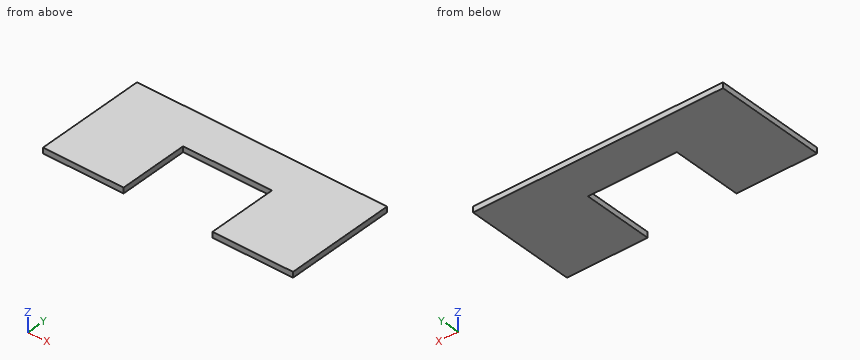
Autodesk Fusion 360 part; units mm, degrees
sketch "Sorting Mechanism Top Panel" plane through (0, 0, 0) normal (0, 0, 1) x (1, 0, 0)
  line L0 (0, 0) -> (270, 0)
  line L1 (270, 0) -> (270, 120)
  line L2 (270, 120) -> (0, 120)
  line L3 (0, 120) -> (0, 0)
  dimension "d1" = 270
  dimension "d2" = 120
extrude "Extrude1" add sketch "Sorting Mechanism Top Panel" along normal blind 6
sketch "Smartie Hopper Hole" plane through (0, 0, 6) normal (0, 0, 1) x (-1, 0, 0)
  line L0 (0, -120) -> (0, 0)
  line L1 (0, 0) -> (-270, 0)
  line L2 (-270, 0) -> (-270, -120)
  line L3 (-270, -120) -> (0, -120)
  line L4 (-87, -76) -> (-183, -76)
  line L5 (-183, -76) -> (-183, 0)
  line L6 (-183, 0) -> (-87, 0)
  line L7 (-87, 0) -> (-87, -76)
  dimension "d7" = 96
  dimension "d9" = 76
  dimension "d10" = 87
  dimension "d11" = 87
extrude "Extrude2" cut sketch "Smartie Hopper Hole" against normal blind 6 contours L1 L4 L5 L6 L7
equation "d3 = MDF_thickness"
equation "acrylic_thickness = 3 mm"
equation "MDF_thickness = 6 mm"
equation "d7 = smarties_hopper_width + 2 * acrylic_thickness"
equation "smarties_hopper_width = 90 mm"
equation "d9 = smarties_hopper_depth + 2 * acrylic_thickness"
equation "d10 = ( 270 mm - ( smarties_hopper_width + 2 * acrylic_thickness ) ) / 2"
equation "smarties_hopper_depth = 70 mm"
The model under review builds one solid part; all positions refer to its coordinate system, in mm. Round coordinates to 2 decimals unless told otherwise and drop trailing zeros. Write each loop counter-clockwise with the first axis right and the second up, starting at its lowest first coordinate (ties: lowest second). Pieces come first, ordered by that corner, then holes. Notation, with made-up numbers: M -10,0 L 39,0 A18 cw 39,30 Z; hole C -24,82.5 d7. An arc over 180 degrees is marked long. Answer as CSV lines item,"result". Start each with the question number.
Q1. Clearance check with a flat-ended pin moving along its axis: P1, Ø3, axis at x = 141.5, z = 1.5, coming from the -Y side. State where the tip first meets the part, or that it passes through.
Q2. Consider section B-B, the plane z = 3. Give the boundary of the cut face in (x, y), then the cut area to 3 significant figures.
Q3. Wall thickness on line 1 along X through (y, z) = (25.5, 4.7); line 2 along Y through (x, z) = (128, 4.6): over which ranges is each line inside the solid? List them lowest first.
Q4. Consider section C-C, the plane x = 153. Give the boundary of the cut face in (y, z), then the cut area to 3 significant figures.
Q5. Consider section A-A, the plane y = 25.5. Give the boundary of the cut face in (x, z), then the cut area to 3 significant figures.
Result set:
1,P1,"stops at y = 76"
2,outline,"M 0,0 L 87,0 L 87,76 L 183,76 L 183,0 L 270,0 L 270,120 L 0,120 Z"
2,area,"25,100 mm²"
3,line 1,"x = 0 to 87, 183 to 270"
3,line 2,"y = 76 to 120"
4,outline,"M 76,0 L 120,0 L 120,6 L 76,6 Z"
4,area,"264 mm²"
5,outline,"M 0,0 L 87,0 L 87,6 L 0,6 Z; M 183,0 L 270,0 L 270,6 L 183,6 Z"
5,area,"1,040 mm²"
